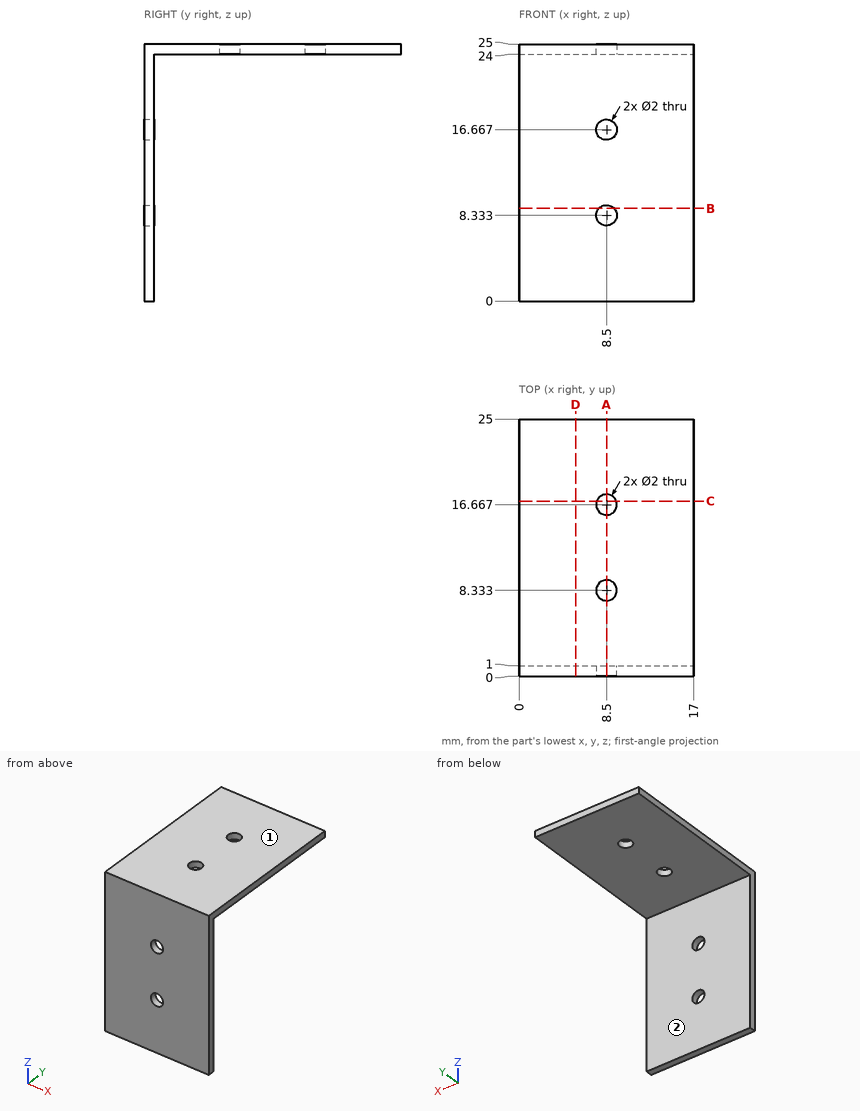
For this review, use the dimensioned drawing (mm, ordinates from the lowest corner) and the shaded views. A direction names the side the tool comes from. Round coordinates to 2 decimals unless told otherwise and drop trailing zeros. Write each loop counter-clockwise with the first axis right and the second up, starting at its lowest first coordinate (ties: lowest second). Pieces come first, ordered by that corner, then holes. Notation, with made-up numbers: (-34, 40) -> (-20, 40) arc R21 cw to (-20, 49) -> close; hole circle Ø4 at (-24.5, -18.5). An arc over 180 degrees is marked (long way). Answer in a Markdown table with one row per item.
Q1. For the marked faces 1 and 2, list the 3-axis set-ups (+Z, -Z, +X, -X, +Y, -Y) from which the entire face can be reached by the end or side of a thin tool; tool diameter is ignored.
The answers:
| item | result |
|---|---|
| face 1 | +Z, +X, -X, +Y, -Y |
| face 2 | -Z, +X, -X, +Y |
Q2. Clearance check with flat-ended pins moving along their axes: pin 1 Ø8.5 at (x, y) = (9, 19) entering from -Z; pin 2 Ø8.5 at (x, z) = (6, 8.5) entering from +Y; pin 3 Ø10 at (x, z) = (3, 14.5) entering from -Y. State where each tip first meets the part, or that it passes through.
The answers:
| item | result |
|---|---|
| pin 1 | z = 24 |
| pin 2 | y = 1 |
| pin 3 | y = 0 |
Q3. Take a section at C-C, the plane y = 17. State the section outline as (x, z) points, then the cut area to 3 significant figures.
The answers:
| item | result |
|---|---|
| outline | (0, 24) -> (7.56, 24) -> (7.56, 25) -> (0, 25) -> close; (9.44, 24) -> (17, 24) -> (17, 25) -> (9.44, 25) -> close |
| area | 15.1 mm² |
Q4. Take a section at A-A, the plane x = 8.5. State the section outline as (y, z) points.
The answers:
| item | result |
|---|---|
| outline | (0, 0) -> (1, 0) -> (1, 7.33) -> (0, 7.33) -> close; (0, 9.33) -> (1, 9.33) -> (1, 15.67) -> (0, 15.67) -> close; (0, 17.67) -> (1, 17.67) -> (1, 24) -> (7.33, 24) -> (7.33, 25) -> (0, 25) -> close; (9.33, 24) -> (15.67, 24) -> (15.67, 25) -> (9.33, 25) -> close; (17.67, 24) -> (25, 24) -> (25, 25) -> (17.67, 25) -> close |
Q5. Take a section at B-B, the plane z = 9. State the section outline as (x, y) points (1 decimal).
The answers:
| item | result |
|---|---|
| outline | (0, 0) -> (7.8, 0) -> (7.8, 1) -> (0, 1) -> close; (9.2, 0) -> (17, 0) -> (17, 1) -> (9.2, 1) -> close |
Q6. To check wall thickness, follow L1, parallel to Y at x = 8.5, z = 24.35; L2, parallel to Z at x = 1, y = 22.25. State the ranges of each line that lie inside material, in increasing order. Write a range as [from, to].
The answers:
| item | result |
|---|---|
| L1 | [0, 7.33], [9.33, 15.67], [17.67, 25] |
| L2 | [24, 25] |
Q7. Take a section at D-D, the plane x = 5.5. State the section outline as (y, z) points.
The answers:
| item | result |
|---|---|
| outline | (0, 0) -> (1, 0) -> (1, 24) -> (25, 24) -> (25, 25) -> (0, 25) -> close |
